Study the drawing (mm; zero at the part's minimum x, y, z) and answer. A direction names the side the tool comes from. Coordinates: 2 decimals unless noted, no trailing zeros. Order: outer loops, then holes, each group sorted by start corner. A loop starts at its lowest first (then second) coordinate and runs counter-clockwise, first axis right, second up. Notation, with made-up numbers: (-31.5, 34) - (-15.5, 34) arc R17 cw to (-15.5, 46) - close; hole circle Ø10 at (67, 38.5). An arc over 180 degrees is marked (long way). Write item = value, one per line.
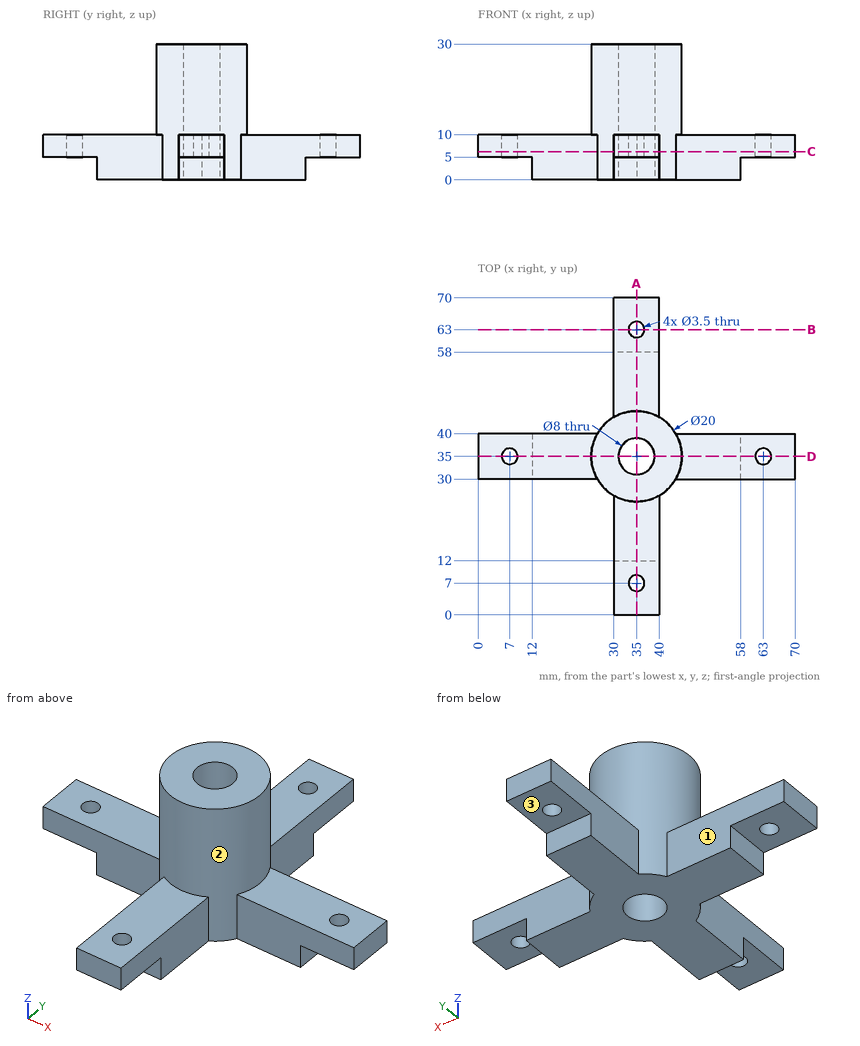
1) Straight lines are drawn through the part: line 1 along Y through (x, z) = (35, 8.95); line 2 along Y through (x, z) = (48, 7.25). For each, find the intervals that lie inside material, in ascending order. Write a range as from..to.
Returned:
line_1 = 0..5.25, 8.75..31, 39..61.25, 64.75..70
line_2 = 30..40
2) The part is cut by section A-A (x = 35). Determine the outline of the cut face in (y, z), and give its area (3 significant figures).
Returned:
outline = (0, 5) - (5.25, 5) - (5.25, 10) - (0, 10) - close; (8.75, 5) - (12, 5) - (12, 0) - (31, 0) - (31, 30) - (25, 30) - (25, 10) - (8.75, 10) - close; (39, 0) - (58, 0) - (58, 5) - (61.25, 5) - (61.25, 10) - (45, 10) - (45, 30) - (39, 30) - close; (64.75, 5) - (70, 5) - (70, 10) - (64.75, 10) - close
area = 705 mm^2
3) For the marked faces 1, 2 and 3, determine the directions among +Z, -Z, +X, -X, +Y, -Y from which every point of the face is accessible in a straight line to the end or side of a thin tool.
Returned:
face_1 = +Z, -Z, -X, +Y
face_2 = +Z
face_3 = -Z, +X, -X, +Y
4) The part is cut by section C-C (z = 6.25). Determine the outline of the cut face in (x, y).
Returned:
outline = (0, 30) - (26.34, 30) arc R10 ccw to (30, 26.34) - (30, 0) - (40, 0) - (40, 26.34) arc R10 ccw to (43.66, 30) - (70, 30) - (70, 40) - (43.66, 40) arc R10 ccw to (40, 43.66) - (40, 70) - (30, 70) - (30, 43.66) arc R10 ccw to (26.34, 40) - (0, 40) - close; hole circle Ø3.5 at (7, 35); hole circle Ø8 at (35, 35); hole circle Ø3.5 at (35, 7); hole circle Ø3.5 at (35, 63); hole circle Ø3.5 at (63, 35)
5) The part is cut by section B-B (y = 63). Determine the outline of the cut face in (x, z), and give its area (3 significant figures).
Returned:
outline = (30, 5) - (33.25, 5) - (33.25, 10) - (30, 10) - close; (36.75, 5) - (40, 5) - (40, 10) - (36.75, 10) - close
area = 32.5 mm^2
6) Flat-ended cylindrical pins translate along their axes: pin 1 Ø2 at (x, z) = (17.5, 5.5) entering from -Y; pin 2 Ø11 at (x, y) = (7.5, 37.5) entering from -Z; pin 3 Ø8 at (x, y) = (34, 64.5) entering from -Z; pin 4 Ø8 at (y, z) = (34.5, 23) entering from +X. Find the tip coordinate at first contact, or state that the pin passes through.
Returned:
pin_1 = 30
pin_2 = 0
pin_3 = 5
pin_4 = 45
